```python
from build123d import *

# Parameters (mm, degrees)
F1_DEPTH     = 64.135
F3_DEPTH     = 76.2
F5_DEPTH     = 3.175
F6_R         = 0.79375
F7_T1_DEPTH  = 3.6287733717
F7_T6_DEPTH  = 4.4225233717
F7_T8_DEPTH  = 4.8762967434
F7_T13_DEPTH = 63.7950233717
F7_T18_DEPTH = 4.4225233717
F7_T23_DEPTH = 6.4637967434
F7_T25_DEPTH = 4.8762967434


# Not quite as in the source:
# - a fillet or chamfer that OpenCascade refuses, or shapes differently, is made with other operations: its cross-section is extruded or revolved along the edge and cut away or added


with BuildPart() as f1:
    # F0 (on Front) → F1 (new body)
    with BuildSketch(Plane.XZ):
        with BuildLine():
            ThreePointArc((10.7345036748, 23.0202178716), (24.8808005482, -5.1093800095), (0.79375, -25.3875946269))
            Line((0.79375, -25.3875946269), (0.79375, -28.563973567))
            ThreePointArc((0.79375, -28.563973567), (2.3849591955, -28.4752979727), (3.96875, -28.2980502586))
            ThreePointArc((3.96875, -28.2980502586), (26.4678099831, -10.7696638619), (22.5988525327, 17.4877811401))
            Line((22.5988525327, 17.4877811401), (10.7345036748, 23.0202178716))
        make_face()
        with BuildLine():
            Line((-1.1298448363, 28.5526544413), (10.7345036748, 23.0202178716))
            Line((10.7345036748, 23.0202178716), (22.5988525327, 17.4877811401))
            ThreePointArc((22.5988525327, 17.4877811401), (17.8402275241, 22.3216689987), (12.0763169886, 25.8977449403))
            ThreePointArc((12.0763169886, 25.8977449403), (5.6319134635, 28.0144993841), (-1.1298448363, 28.5526544413))
        make_face()
        with BuildLine():
            ThreePointArc((-0.79375, -25.3875946269), (-24.708980627, 5.8844096028), (10.7345036748, 23.0202178716))
            Line((10.7345036748, 23.0202178716), (-1.1298448363, 28.5526544413))
            ThreePointArc((-1.1298448363, 28.5526544413), (-28.5394389143, 1.4251496253), (-3.96875, -28.2980502586))
            ThreePointArc((-3.96875, -28.2980502586), (-2.3849591955, -28.4752979727), (-0.79375, -28.563973567))
            Line((-0.79375, -28.563973567), (-0.79375, -25.3875946269))
        make_face()
        with BuildLine():
            ThreePointArc((3.96875, -28.2980502586), (2.3849591955, -28.4752979727), (0.79375, -28.563973567))
            Line((0.79375, -28.563973567), (0.79375, -34.925))
            Line((0.79375, -34.925), (3.96875, -34.925))
            Line((3.96875, -34.925), (3.96875, -28.2980502586))
        make_face()
        with BuildLine():
            ThreePointArc((12.0763169886, 25.8977449403), (17.8402275241, 22.3216689987), (22.5988525327, 17.4877811401))
            Line((22.5988525327, 17.4877811401), (40.6476504402, 9.0714884554))
            Line((40.6476504402, 9.0714884554), (41.9894634213, 11.9490156792))
            Line((41.9894634213, 11.9490156792), (12.0763169886, 25.8977449403))
        make_face()
        with BuildLine():
            Line((-28.413002932, 41.275), (-1.1298448363, 28.5526544413))
            ThreePointArc((-1.1298448363, 28.5526544413), (5.6319134635, 28.0144993841), (12.0763169886, 25.8977449403))
            Line((12.0763169886, 25.8977449403), (-27.0711899509, 44.1525272238))
            Line((-27.0711899509, 44.1525272238), (-28.413002932, 41.275))
        make_face()
        with BuildLine():
            Line((-0.79375, -34.925), (-0.79375, -28.563973567))
            ThreePointArc((-0.79375, -28.563973567), (-2.3849591955, -28.4752979727), (-3.96875, -28.2980502586))
            Line((-3.96875, -28.2980502586), (-3.96875, -34.925))
            Line((-3.96875, -34.925), (-0.79375, -34.925))
        make_face()
    extrude(amount=F1_DEPTH)

    # F2 (on face) → F3 (join, through all)
    with BuildSketch(Plane(origin=(-39.1475067802, 0, 18.2547822093), x_dir=(0, -1, 0), z_dir=(-0.906307787, 0, 0.4226182617))):
        Polygon((0, 31.75), (0, 28.575), (1.5875, 28.575), (1.5875, 30.1625), (3.175, 30.1625), (3.175, 31.75), align=None)
        Polygon((62.5475, 30.1625), (62.5475, 28.575), (64.135, 28.575), (64.135, 31.75), (60.96, 31.75), (60.96, 30.1625), align=None)
    extrude(amount=-F3_DEPTH)

    # F4 (on face) → F5 (join)
    with BuildSketch(Plane(origin=(29.913146592, 0, -13.9487293354), x_dir=(0, 1, 0), z_dir=(0.906307787, 0, -0.4226182617))):
        Polygon((-3.175, 31.75), (-60.96, 31.75), (-60.96, 30.1625), (-62.5475, 30.1625), (-62.5475, 28.575), (-1.5875, 28.575), (-1.5875, 30.1625), (-3.175, 30.1625), align=None)
    extrude(amount=-F5_DEPTH)

    # F6
    f6_edges = [f1.edges().sort_by_distance(p)[0] for p in [
        (-28.539439, 0, 1.42515),
        (-28.539439, -64.135, 1.42515),
        (-1.129845, -32.0675, 28.552654),
        (-3.96875, -32.0675, -28.29805),
        (22.598853, -32.0675, 17.487781),
        (3.96875, -32.0675, -28.29805),
        (26.46781, 0, -10.769664),
        (26.46781, -64.135, -10.769664),
        (41.989463, 0, 11.949016),
        (40.64765, -32.0675, 9.071488),
        (41.989463, -64.135, 11.949016),
        (3.96875, -64.135, -31.611525),
        (31.623251, -64.135, 13.279635),
        (-14.771424, -64.135, 34.913827),
        (-3.96875, -64.135, -31.611525),
        (-3.96875, 0, -31.611525),
        (-14.771424, 0, 34.913827),
        (31.623251, 0, 13.279635),
        (3.96875, 0, -31.611525),
    ]]
    fillet(f6_edges, radius=F6_R)

    # F7: chamfer of 0.79375 on 7 edges, made by hand

    # F7_s2 → F7_t1 (cut)
    with BuildSketch(Plane.XZ.offset(1.5875)):
        Polygon((-26.0648302152, 46.3106726417), (-25.6809016545, 45.2558375905), (-26.4002834604, 45.5912908358), align=None)
    extrude(amount=F7_T1_DEPTH, mode=Mode.SUBTRACT)


with BuildPart() as f7_tool4:
    # F7_s5 → F7_t6 (new body)
    with BuildSketch(Plane(origin=(12.0763168292, 0, 25.8977450146), x_dir=(0, 1, 0), z_dir=(0.4226182617, 0, 0.906307787))):
        Polygon((-0.79375, 43.1944945637), (-1.5875, 42.4007445637), (-1.5875, 43.1944945637), align=None)
    extrude(amount=F7_T6_DEPTH)

    split(bisect_by=Plane(origin=(-8.131860996, 0, -2.9597553517), x_dir=(0, 1, 0), z_dir=(-0.9396926208, 0, -0.3420201433)), keep=Keep.TOP)


with BuildPart() as f1_1:
    add(f1.part)

    # F7_t3: cut F7_tool4
    add(f7_tool4.part, mode=Mode.SUBTRACT)

    # F7_s9 → F7_t8 (cut)
    with BuildSketch(Plane(origin=(12.2199971609, 0, 26.2058684802), x_dir=(0, 1, 0), z_dir=(0.4226182617, 0, 0.906307787))):
        Polygon((-2.38125, 43.1944945637), (-3.175, 42.4007445637), (-3.175, 43.1944945637), align=None)
    extrude(amount=F7_T8_DEPTH, mode=Mode.SUBTRACT)


with BuildPart() as f7_tool11:
    # F7_s12 → F7_t13 (new body)
    with BuildSketch(Plane.XZ.offset(62.5475)):
        Polygon((-27.4066431962, 43.4331454179), (-26.351808145, 43.8170739786), (-27.0711899509, 44.1525272238), align=None)
    extrude(amount=-F7_T13_DEPTH)

    split(bisect_by=Plane(origin=(-19.9334442931, -21.9941222818, 9.2951177273), x_dir=(0.7409656453, -0.6715429342, 0), z_dir=(-0.6408563821, -0.7071067812, 0.2988362387)), keep=Keep.TOP)


with BuildPart() as f1_2:
    add(f1_1.part)

    # F7_t10: cut F7_tool11
    add(f7_tool11.part, mode=Mode.SUBTRACT)


with BuildPart() as f7_tool16:
    # F7_s17 → F7_t18 (new body)
    with BuildSketch(Plane(origin=(12.7472233198, 0, 27.3365086265), x_dir=(0, 1, 0), z_dir=(-0.4226182617, 0, -0.906307787))):
        Polygon((-63.34125, -43.1944945637), (-62.5475, -42.4007445637), (-62.5475, -43.1944945637), align=None)
    extrude(amount=F7_T18_DEPTH)

    split(bisect_by=Plane(origin=(-17.1651120978, 0, 47.160757891), x_dir=(0, 1, 0), z_dir=(-0.3420201433, 0, 0.9396926208)), keep=Keep.TOP)


with BuildPart() as f1_3:
    add(f1_2.part)

    # F7_t15: cut F7_tool16
    add(f7_tool16.part, mode=Mode.SUBTRACT)


with BuildPart() as f7_tool21:
    # F7_s22 → F7_t23 (new body)
    with BuildSketch(Plane.XZ.offset(58.9187266283)):
        Polygon((-26.0648302152, 46.3106726417), (-25.6809016545, 45.2558375905), (-26.4002834604, 45.5912908358), align=None)
    extrude(amount=F7_T23_DEPTH)

    split(bisect_by=Plane(origin=(9.1295806677, -10.0733777182, -4.2571933811), x_dir=(-0.7409656453, -0.6715429342, 0), z_dir=(-0.6408563821, 0.7071067812, 0.2988362387)), keep=Keep.TOP)


with BuildPart() as f1_4:
    add(f1_3.part)

    # F7_t20: cut F7_tool21
    add(f7_tool21.part, mode=Mode.SUBTRACT)

    # F7_s26 → F7_t25 (cut)
    with BuildSketch(Plane(origin=(14.2808092144, 0, 30.6252941907), x_dir=(0, 1, 0), z_dir=(-0.4226182617, 0, -0.906307787))):
        Polygon((-61.75375, -43.1944945637), (-60.96, -42.4007445637), (-60.96, -43.1944945637), align=None)
    extrude(amount=F7_T25_DEPTH, mode=Mode.SUBTRACT)


solid = f1_4.part
```
Input: part model. Units: mm. Frame: model coordinates. A direction names the side the tool comes from. Give positions to 0.01 mm unless a question says otherwise; leave off trailing zeros. Put each result on its own line as item: value.
Item 1: Access query for faces 1 (the flat face through (6, -62.548, 29)), 2 (the flat face through (-16.277, -31.63, 35.616)), 3 (the flat face through (0.794, -32, -30)), 4 (the cylindrical face through (-15.83, -63.91, 35.67)). Directions: +Z, -Z, +X, -X, +Y, -Y. A direction counts if a zero-diameter tool reaches every point of the face in a straight line with its end or side. Return the directions, or none.
Found:
face 1: none
face 2: -X, +Y, -Y
face 3: -Z, +Y, -Y
face 4: -X, -Y
Item 2: Contact query for flat-ended pins moving along their axis: pin 1 (6 mm diameter, centred on x = 6, y = -26, fed in from +Z); pin 2 (10.5 mm diameter, centred on y = -38.5, z = -28.5, fed in from +X); pin 3 (6 mm diameter, centred on x = 15.5, y = -25, fed in from +Z). Output: stop coordinate, or through.
Found:
pin 1: stops at z = 30.13
pin 2: stops at x = 16.61
pin 3: stops at z = 25.7
Item 3: Ray query, L1, parallel to X at y = -19, z = 0 (3 decimals); L2, parallel to Y at x = 31.5, z = 19 (3 decimals); L3, parallel to Z at x = -22.5, y = -56.5. Return the intervals inside material, ascending. Write a range as from..to.
Found:
L1: x = -28.575..-25.4, 25.4..28.575
L2: y = -64.135..-60.96, -3.175..0
L3: z = -17.61..-11.79, 11.79..17.61, 38.52..42.02
Item 4: Draft query along Y for faces 5 (the cylindrical face through (-28.56, -31.63, 0.88)), 6 (the flat face through (6.593, -61.743, 30.206)), 7 (the flat face through (10, -64.135, 24)). Return one class per face: +Y half, -Y half, draft (parallel to the pull), parting line (faces both ways), or undercut.
Found:
face 5: draft
face 6: undercut
face 7: -Y half
